Part model, mm, in its own coordinate system. Face numbers are marked on the shaded views. A direction names the side the tool comes from. Round coordinates to 2 decimals unless told otherwise and drop trailing zeros. Write each loop counter-clockwise with the first axis right and the second up, starting at its lowest first coordinate (ties: lowest second). Pieces come first, ordered by that corner, then holes.
1) Pull direction X, two halves, no side cores. Call the marked faces 3, 4 and 5: +X half, -X half, draft (parallel to the pull), parting line (faces both ways), or undercut.
2) Which spindle directions (+Z, -Z, +X, -X, +Y, -Y) get a long thin tool onto all of the face, cutting with end or side? Do the marked faces 1 and 2. Say none if no direction does.
3) Saw through at C-C on y = 20.25. Write the cut outline in (x, z), and give its area (3 significant figures).
4) Flat gauge pins, fed straight in: pin 1 (1 mm diameter, centred on x = 6, y = 19, fed in from -Z); pin 2 (1 mm diameter, centred on x = 9.5, y = 18.5, fed in from -Z). Where does each tip first touch, or does it go through?
5) Drill centre lines: L1, parallel to X at y = 15.5, z = -0.25; L2, parallel to Z at x = -1, y = 20.75; L3, parallel to Z at x = 12, y = 16. Where is each one in solid material? Low to high.
6) Saw through at A-A on y = 18.25. Write the cut outline in (x, z), and give its area (3 significant figures).
7) Saw through at D-D on y = 16. Write the cut outline in (x, z), and give its area (3 significant figures).
```python
from build123d import *

# Parameters (mm, degrees)
SKETCH2_R           = 2.055531292
BOSS_EXTRUDE1_DEPTH = 10
SKETCH3_W           = 13.058934706
SKETCH3_H           = 7.734398283
BOSS_EXTRUDE2_DEPTH = 13.356191657


with BuildPart() as part:
    # Sketch2 → Boss-Extrude1 (new body)
    with BuildSketch(Plane(origin=(6.678095828, 0, 0), x_dir=(0, 0, -1), z_dir=(1, 0, 0))):
        with BuildLine():
            Line((2.069151562, 21.444166214), (-3.368651258, 21.444166214))
            Line((-3.368651258, 21.444166214), (-13.95384316, 21.444166214))
            Line((-13.95384316, 21.444166214), (-13.95384316, 13.709767931))
            Line((-13.95384316, 13.709767931), (-3.368651258, 13.709767931))
            Line((-3.368651258, 13.709767931), (2.069151562, 13.709767931))
            ThreePointArc((2.069151562, 13.709767931), (5.936350704, 17.576967072), (2.069151562, 21.444166214))
        make_face()
        with Locations(Location((2.069151562, 17.576967072, 0), (0, 0, 90))):
            Circle(SKETCH2_R, mode=Mode.SUBTRACT)
    extrude(amount=BOSS_EXTRUDE1_DEPTH)


with BuildPart() as body_2:
    # Mirror2: mirrored copy
    add(part.part.mirror(Plane(origin=(0, 0, 0), x_dir=(0, 0, 1), z_dir=(1, 0, 0))))


with BuildPart() as part_1:
    add(part.part)

    add(body_2.part)  # Boss-Extrude2 merges body 2
    # Sketch3 → Boss-Extrude2 (add)
    with BuildSketch(Plane.ZY.offset(-6.678095828)):
        with Locations((7.424375807, 17.576967073)):
            Rectangle(SKETCH3_W, SKETCH3_H)
    extrude(amount=BOSS_EXTRUDE2_DEPTH)


solid = part_1.part
```
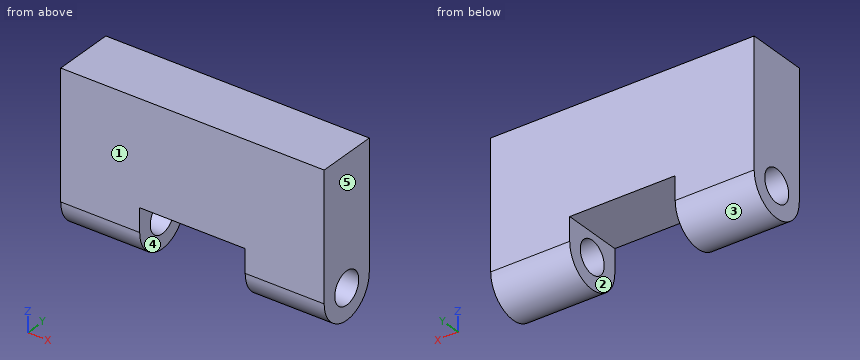
Completed:
1. face 3: draft
1. face 4: undercut
1. face 5: +X half
2. face 1: +Z, -Z, +X, -X, -Y
2. face 2: -Z, +Y, -Y
3. outline: (-16.68, -4.86) - (-6.68, -4.86) - (-6.68, 0.89) - (6.68, 0.89) - (6.68, -4.86) - (16.68, -4.86) - (16.68, 13.95) - (-16.68, 13.95) - close
3. area: 551 mm2
4. pin 1: stops at z = 0.89
4. pin 2: stops at z = -5.91
5. L1: x = -16.68 to -6.68, 6.68 to 16.68
5. L2: z = 0.89 to 13.95
5. L3: z = -5.6 to -3.39, -0.75 to 13.95
6. outline: (-16.68, -5.88) - (-6.68, -5.88) - (-6.68, -4.01) - (-16.68, -4.01) - close; (-16.68, -0.13) - (-6.68, -0.13) - (-6.68, 0.89) - (6.68, 0.89) - (6.68, -0.13) - (16.68, -0.13) - (16.68, 13.95) - (-16.68, 13.95) - close; (6.68, -5.88) - (16.68, -5.88) - (16.68, -4.01) - (6.68, -4.01) - close
6. area: 493 mm2
7. outline: (-16.68, -5.6) - (-6.68, -5.6) - (-6.68, -3.39) - (-16.68, -3.39) - close; (-16.68, -0.75) - (-6.68, -0.75) - (-6.68, 0.89) - (6.68, 0.89) - (6.68, -0.75) - (16.68, -0.75) - (16.68, 13.95) - (-16.68, 13.95) - close; (6.68, -5.6) - (16.68, -5.6) - (16.68, -3.39) - (6.68, -3.39) - close
7. area: 513 mm2
